Study the drawing (mm; zero at the part's minimum x, y, z) and answer. A direction names the side the tool comes from. Coordinates: 2 decimals unless noted, no trailing zeros. Loops run counter-clockwise (first coordinate to the right, second up) from the corner with the lowest first, then second, coordinate; pieces in that order, holes last. Notation, with made-up numbers: (-3.75, 6) -> (38.25, 6) arc R25 ccw to (38.25, 34) -> close; hole circle Ø5 at (-10, 28.25). An arc over 180 degrees is marked (long way). One line per question, with ' | ' between items.
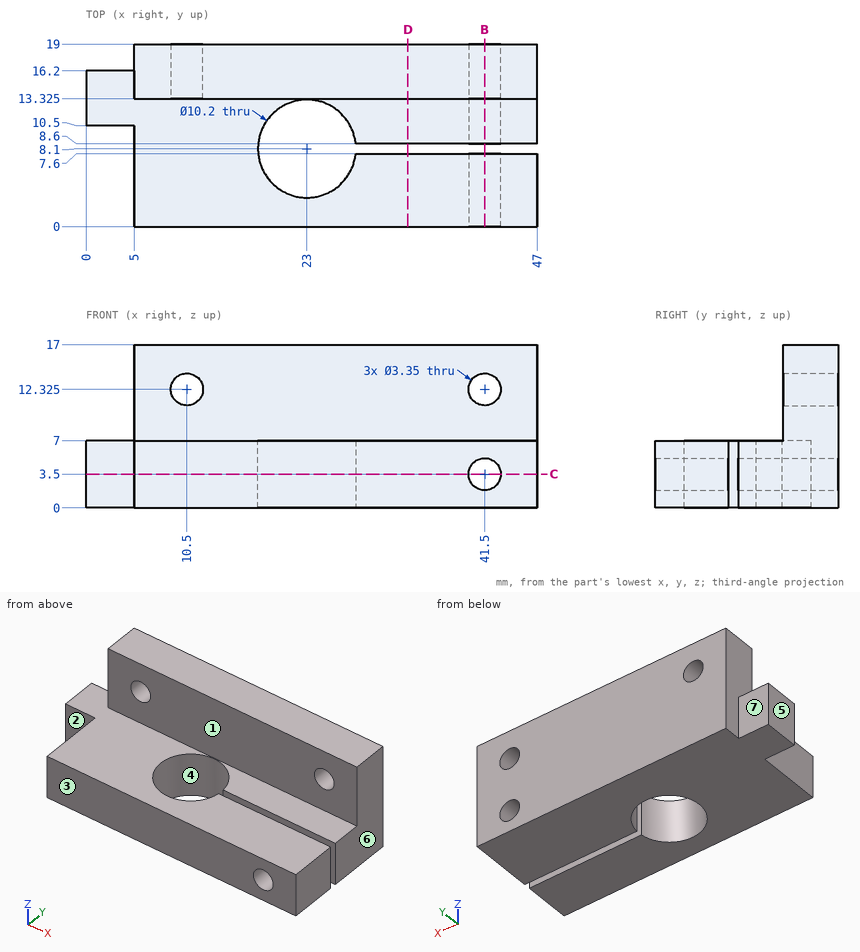
1) For the marked faces 1, 2 and 3, determine the directions among +Z, -Z, +X, -X, +Y, -Y from which every point of the face is accessible in a straight line to the end or side of a thin tool.
Check values:
face 1: +Z, +X, -X, -Y | face 2: +Z, -Z, -X, -Y | face 3: +Z, -Z, +X, -X, -Y
2) Find the intervals of material crossed by line 1 along Y through (x, z) = (23, 4.75); line 2 along Y through (x, z) = (36.5, 2); line 3 along X through (y, z) = (9, 3), in increasing order.
Check values:
line 1: y = 0 to 3, 13.2 to 19 | line 2: y = 0 to 7.6, 8.6 to 19 | line 3: x = 5 to 17.98, 28.02 to 39.9, 43.1 to 47
3) The mould has two halves that part along X. Classify the marked faces 4, 5, 6 and 7: released by +X, released by -X, zero draft, split by the parting line, or undercut.
Check values:
face 4: undercut | face 5: released by -X | face 6: released by +X | face 7: zero draft
4) Find section B-B (x = 41.5). State how many separate pieces and enclosed holes the cut face has.
Check values:
separate pieces: 5 | enclosed holes: 0
5) Flat-ended cylindrical pins translate along their axes: pin 1 (10 mm diameter, centred on x = 18.5, y = 4, fed in from +Z); pin 2 (2 mm diameter, centred on x = 41.5, z = 12.325, fed in from -Y); pin 3 (3.5 mm diameter, centred on y = 4.5, z = 2, fed in from -X); pin 4 (4.5 mm diameter, centred on x = 10.5, z = 12.325, fed in from -Y) (1 decimal). Find the tip coordinate at first contact, or state that the pin passes through.
Check values:
pin 1: stops at z = 7 | pin 2: passes through | pin 3: stops at x = 5 | pin 4: stops at y = 13.3
6) Find section C-C (z = 3.5). Write down the section's boundary in (x, y) (1 decimal).
Check values:
outline: (0, 10.5) -> (5, 10.5) -> (5, 0) -> (39.8, 0) -> (39.8, 7.6) -> (28.1, 7.6) arc R5.1 cw (long way) to (28.1, 8.6) -> (39.8, 8.6) -> (39.8, 19) -> (5, 19) -> (5, 16.2) -> (0, 16.2) -> close; (43.2, 0) -> (47, 0) -> (47, 7.6) -> (43.2, 7.6) -> close; (43.2, 8.6) -> (47, 8.6) -> (47, 19) -> (43.2, 19) -> close
7) Find section D-D (x = 33.5). Write down the section's boundary in (y, z) (1 decimal), plus the area to 3 significant figures.
Check values:
outline: (0, 0) -> (7.6, 0) -> (7.6, 7) -> (0, 7) -> close; (8.6, 0) -> (19, 0) -> (19, 17) -> (13.3, 17) -> (13.3, 7) -> (8.6, 7) -> close | area: 183 mm^2
